The model under review builds one solid part; all positions refer to its coordinate system, in mm. A direction names the side the tool comes from. Coordinates: 2 decimals unless noted, no trailing zeros. Order: outer loops, then holes, each group sorted by start corner. A loop starts at its lowest first (then second) coordinate and runs counter-clockwise, first axis right, second up. Notation, with made-up numbers: (42.5, 70.5) - (76.5, 70.5) arc R26 cw to (76.5, 95.5) - close; hole circle Ø9 at (45, -30). An arc over 180 degrees is marked (long way). Answer in a Markdown table with one row per item.
Autodesk Inventor part; units mm, degrees
ref_plane "YZ Plane" through (0, 0, 0) normal (1, 0, 0) x (0, 1, 0)
ref_plane "XZ Plane" through (0, 0, 0) normal (0, 1, 0) x (-1, 0, 0)
ref_plane "XY Plane" through (0, 0, 0) normal (0, 0, 1) x (1, 0, 0)
sketch "스케치3" plane through (0, 0, 0) normal (0, 1, 0) x (-1, 0, 0)
  line L0 (35.7919, -14.8255) -> (14.8255, -35.7919)
  line L1 (14.8255, -35.7919) -> (-14.8255, -35.7919)
  line L2 (-14.8255, -35.7919) -> (-35.7919, -14.8255)
  line L3 (-35.7919, -14.8255) -> (-35.7919, 14.8255)
  line L4 (-35.7919, 14.8255) -> (-14.8255, 35.7919)
  line L5 (-14.8255, 35.7919) -> (14.8255, 35.7919)
  line L6 (14.8255, 35.7919) -> (35.7919, 14.8255)
  line L7 (35.7919, 14.8255) -> (35.7919, -14.8255)
  line L8 (13.5, -32.5919) -> (-13.5, -32.5919)
  line L9 (-13.5, -32.5919) -> (-32.5919, -13.5)
  line L10 (-32.5919, -13.5) -> (-32.5919, 13.5)
  line L11 (-32.5919, 13.5) -> (-13.5, 32.5919)
  line L12 (-13.5, 32.5919) -> (13.5, 32.5919)
  line L13 (13.5, 32.5919) -> (32.5919, 13.5)
  line L14 (32.5919, 13.5) -> (32.5919, -13.5)
  line L15 (32.5919, -13.5) -> (13.5, -32.5919)
  point P0 (0, 0)
  point P1 (0, 0)
  point P2 (0, 0)
  point P3 (0, 0)
  dimension "d66" = 27
  dimension "d67" = 3.2
extrude "돌출2" add sketch "스케치3" along normal blind 3.7 contours L0 L1 L2 L3 L4 L5 L6 L7 | L8 L9 L10 L11 L12 L13 L14 L15
sketch "스케치4" plane through (0, 3.7, 0) normal (0, 1, 0) x (1, 0, 0)
  line L0 (13.5, -32.5919) -> (-13.5, -32.5919)
  line L1 (-13.5, -32.5919) -> (-32.5919, -13.5)
  line L2 (-32.5919, -13.5) -> (-32.5919, 13.5)
  line L3 (-32.5919, 13.5) -> (-13.5, 32.5919)
  line L4 (-13.5, 32.5919) -> (13.5, 32.5919)
  line L5 (13.5, 32.5919) -> (32.5919, 13.5)
  line L6 (32.5919, 13.5) -> (32.5919, -13.5)
  line L7 (32.5919, -13.5) -> (13.5, -32.5919)
  line L8 (-14.1627, 34.1919) -> (14.1627, 34.1919)
  line L9 (14.1627, 34.1919) -> (34.1919, 14.1627)
  line L10 (34.1919, 14.1627) -> (34.1919, -14.1627)
  line L11 (34.1919, -14.1627) -> (14.1627, -34.1919)
  line L12 (14.1627, -34.1919) -> (-14.1627, -34.1919)
  line L13 (-14.1627, -34.1919) -> (-34.1919, -14.1627)
  line L14 (-34.1919, -14.1627) -> (-34.1919, 14.1627)
  line L15 (-34.1919, 14.1627) -> (-14.1627, 34.1919)
  line L16 (-13.3343, 32.1919) -> (13.3343, 32.1919)
  line L17 (13.3343, 32.1919) -> (32.1919, 13.3343)
  line L18 (32.1919, 13.3343) -> (32.1919, -13.3343)
  line L19 (32.1919, -13.3343) -> (13.3343, -32.1919)
  line L20 (13.3343, -32.1919) -> (-13.3343, -32.1919)
  line L21 (-13.3343, -32.1919) -> (-32.1919, -13.3343)
  line L22 (-32.1919, -13.3343) -> (-32.1919, 13.3343)
  line L23 (-32.1919, 13.3343) -> (-13.3343, 32.1919)
  line L24 (-14.8255, 35.7919) -> (-35.7919, 14.8255)
  point P0 (0, 0)
  point P1 (0, 0)
  point P2 (0, 0)
  point P3 (0, 0)
  dimension "d7" = 27
  dimension "d99" = 1.6
  dimension "d100" = 2
extrude "돌출3" cut sketch "스케치4" against normal blind 1.2 contours L0 L1 L2 L3 L4 L5 L6 L7 | L8 L9 L10 L11 L12 L13 L14 L15 | L16 L17 L18 L19 L20 L21 L22 L23
sketch "스케치11" plane through (0, 2.5, 0) normal (0, 1, 0) x (1, 0, 0)
  line L0 (-13.3343, 32.1919) -> (13.3343, 32.1919)
  line L1 (13.3343, 32.1919) -> (32.1919, 13.3343)
  line L2 (32.1919, 13.3343) -> (32.1919, -13.3343)
  line L3 (32.1919, -13.3343) -> (13.3343, -32.1919)
  line L4 (13.3343, -32.1919) -> (-13.3343, -32.1919)
  line L5 (-13.3343, -32.1919) -> (-32.1919, -13.3343)
  line L6 (-32.1919, -13.3343) -> (-32.1919, 13.3343)
  line L7 (-32.1919, 13.3343) -> (-13.3343, 32.1919)
  line L8 (-14.1627, 34.1919) -> (14.1627, 34.1919)
  line L9 (-12.0917, 29.1919) -> (12.0917, 29.1919)
  line L10 (12.0917, 29.1919) -> (29.1919, 12.0917)
  line L11 (29.1919, 12.0917) -> (29.1919, -12.0917)
  line L12 (29.1919, -12.0917) -> (12.0917, -29.1919)
  line L13 (12.0917, -29.1919) -> (-12.0917, -29.1919)
  line L14 (-12.0917, -29.1919) -> (-29.1919, -12.0917)
  line L15 (-29.1919, -12.0917) -> (-29.1919, 12.0917)
  line L16 (-29.1919, 12.0917) -> (-12.0917, 29.1919)
  point P0 (0, 0)
  point P1 (0, 0)
  point P2 (0, 0)
  dimension "d70" = 2
  dimension "d71" = 3
extrude "돌출10" add sketch "스케치11" along normal blind 0.6 contours L0 L1 L2 L3 L4 L5 L6 L7 | L9 L10 L11 L12 L13 L14 L15 L16
fillet "모깎기1" radius 1.2 16 edges at (-25.3087, 3.7, 25.3087) (0, 3.7, 35.7919) (25.3087, 3.7, 25.3087) (35.7919, 3.7, 0) (25.3087, 3.7, -25.3087) (0, 3.7, -35.7919) (-25.3087, 3.7, -25.3087) (-35.7919, 3.7, 0) (-25.3087, 0, 25.3087) (0, 0, 35.7919) (25.3087, 0, 25.3087) (35.7919, 0, 0) (25.3087, 0, -25.3087) (0, 0, -35.7919) (-25.3087, 0, -25.3087) (-35.7919, 0, 0)
sketch "스케치16" plane through (0, 0, 0) normal (0, -1, 0) x (1, 0, 0)
  line L0 (-12.5, 10.3) -> (12.5, 10.3)
  line L1 (12.5, 10.3) -> (12.5, 15.3)
  line L2 (12.5, 15.3) -> (-12.5, 15.3)
  line L3 (-12.5, 15.3) -> (-12.5, 10.3)
  line L4 (-12.5, 10.3) -> (12.5, 15.3) construction
  line L5 (12.5, 10.3) -> (-12.5, 15.3) construction
  line L6 (0, 0) -> (12.5, 0)
  line L7 (-12.5, -10.3) -> (12.5, -10.3)
  line L8 (12.5, -10.3) -> (12.5, -15.3)
  line L9 (12.5, -15.3) -> (-12.5, -15.3)
  line L10 (-12.5, -15.3) -> (-12.5, -10.3)
  line L11 (-12.5, -10.3) -> (12.5, -15.3) construction
  line L12 (12.5, -10.3) -> (-12.5, -15.3) construction
  point P0 (0, 12.8)
  point P1 (0, 10.3)
  point P2 (0, -12.8)
  point P3 (0, -10.3)
  dimension "d127" = 5
  dimension "d128" = 25
  dimension "d129" = 10.3
extrude "돌출12" add sketch "스케치16" along normal blind 15
sketch "스케치17" plane through (-12.5, 0, 15.3) normal (0, 0, 1) x (1, 0, 0)
  circle A0 centre (7.5, -7.5) radius 1.25
  line L0 (-1.8284, 0) -> (26.8284, 0)
  line L1 (12.5, 0) -> (12.5, -5.2723)
  circle A1 centre (17.5, -7.5) radius 1.25
  point P0 (12.5, 0)
  dimension "d132" = 2.5
  dimension "d136" = 7.5
  dimension "d137" = 5
extrude "돌출13" cut sketch "스케치17" against normal up to surface (30.6 mm away)
equation "\"d115\" = 55deg"
properties part number "OV-PAM_bottom_2"
Item 1: To check wall thickness, follow line 1 (Z direction, x = 8, y = -13.5); line 2 (Y direction, x = -5, z = 14); line 3 (Y direction, x = -18.5, z = 18.5). State the ranges of each line that lie inside material, in increasing order. Write a range as from..to.
Check values:
| item | result |
|---|---|
| line 1 | -15.3..-10.3, 10.3..15.3 |
| line 2 | -15..-8.75, -6.25..3.1 |
| line 3 | 0..3.1 |
Item 2: We need section B-B, the plane y = -7.5. Write out the cut boundary in (x, z).
Check values:
| item | result |
|---|---|
| outline | (-12.5, -15.3) - (-6.25, -15.3) - (-6.25, -10.3) - (-12.5, -10.3) - close; (-12.5, 10.3) - (-6.25, 10.3) - (-6.25, 15.3) - (-12.5, 15.3) - close; (-3.75, -15.3) - (3.75, -15.3) - (3.75, -10.3) - (-3.75, -10.3) - close; (-3.75, 10.3) - (3.75, 10.3) - (3.75, 15.3) - (-3.75, 15.3) - close; (6.25, -15.3) - (12.5, -15.3) - (12.5, -10.3) - (6.25, -10.3) - close; (6.25, 10.3) - (12.5, 10.3) - (12.5, 15.3) - (6.25, 15.3) - close |
Item 3: We need section C-C, the plane z = 5. Write out the cut boundary in (x, y).
Check values:
| item | result |
|---|---|
| outline | (-35.79, 1.2) arc R1.2 ccw to (-34.59, 0) - (34.59, 0) arc R1.2 ccw to (35.79, 1.2) - (35.79, 2.5) arc R1.2 ccw to (34.59, 3.7) - (34.19, 3.7) - (34.19, 2.5) - (32.19, 2.5) - (32.19, 3.1) - (-32.19, 3.1) - (-32.19, 2.5) - (-34.19, 2.5) - (-34.19, 3.7) - (-34.59, 3.7) arc R1.2 ccw to (-35.79, 2.5) - close |
Item 4: Mouldability with a two-part tool opening along Y and no side actions: class faces 4 (the face through (-22.631, 2.796, 22.895)), 5 (the face through (0, 0, 0)), 6 (the face through (-5.27, -8.72, -12.76)), 7 (the face through (25.21, 3.34, -24.92)) as +Y half, -Y half, draft (parallel to the pull), parting line (faces both ways), or undercut.
Check values:
| item | result |
|---|---|
| face 4 | draft |
| face 5 | -Y half |
| face 6 | undercut |
| face 7 | +Y half |
Item 5: Clearance check with flat-ended pins moving along their axes: pin 1 Ø0.6 at (x, y) = (7, 3) entering from +Z; pin 2 Ø6 at (x, z) = (2.5, -27) entering from +Y; pin 3 Ø0.5 at (y, z) = (3, -6) entering from -X. State where each tip first meets the part, or that it passes through.
Check values:
| item | result |
|---|---|
| pin 1 | z = 35.78 |
| pin 2 | y = 3.1 |
| pin 3 | x = -35.77 |
Item 6: Tool access review of faces 1 (the face through (12.5, -7, -13)), 2 (the face through (22.895, 2.796, 22.631)), 3 (the face through (0, -15, -13)): name each direction out of +Z, -Z, +X, -X, +Y, -Y from which nothing blocks a thin tool from reaching the whole face with its end or side.
Check values:
| item | result |
|---|---|
| face 1 | +Z, -Z, +X, -Y |
| face 2 | +Y |
| face 3 | +Z, -Z, +X, -X, -Y |
Item 7: We need section A-A, the plane x = -5. State how many separate pieces and enclosed holes the cut face has, then the cut area to 3 significant figures.
Check values:
| item | result |
|---|---|
| separate pieces | 3 |
| enclosed holes | 0 |
| area | 345 mm^2 |
Item 8: We need section D-D, the plane y = -1. Write out the cut boundary in (x, z).
Check values:
| item | result |
|---|---|
| outline | (-12.5, -15.3) - (12.5, -15.3) - (12.5, -10.3) - (-12.5, -10.3) - close; (-12.5, 10.3) - (12.5, 10.3) - (12.5, 15.3) - (-12.5, 15.3) - close |
